Input: dimensioned drawing with shaded views. Units: mm. Origin: part minimum x, y, z. A direction names the side the tool comes from. Give positions to 0.01 mm unless a question says otherwise; leave off trailing zeros. Loops run counter-clockwise (first coordinate to the right, second up) from the corner with the lowest first, then second, coordinate; pieces in that order, holes last.
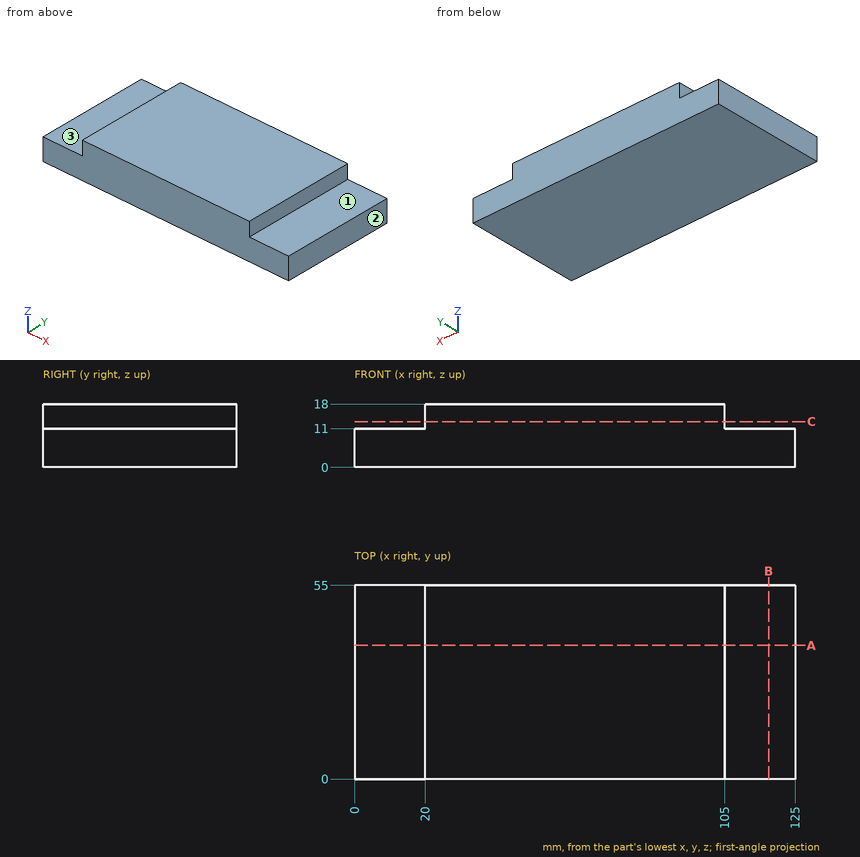
(1) Section C-C, the plane z = 13. Return the cut outline in (x, y), then the cut area to 4 significant figures.
A:
outline: (20, 0) - (105, 0) - (105, 55) - (20, 55) - close
area: 4,675 mm2
(2) Section B-B, the plane x = 117.5. Return the cut outline in (y, z).
A:
outline: (0, 0) - (55, 0) - (55, 11) - (0, 11) - close
(3) Section A-A, the plane y = 38. Return the cut outline in (x, z).
A:
outline: (0, 0) - (125, 0) - (125, 11) - (105, 11) - (105, 18) - (20, 18) - (20, 11) - (0, 11) - close
(4) Ray query, line 1 along X through (y, z) = (50.5, 13.25); line 2 along Z through (x, y) = (16.5, 23). Return the intervals inside material, ascending.
A:
line 1: x = 20 to 105
line 2: z = 0 to 11
(5) Reachability of the marked faces 1, 2 and 3 from +Z, -Z, +X, -X, +Y, -Y: full face, straight path, thin tool, end or side. Return the list, or none.
A:
face 1: +Z, +X, +Y, -Y
face 2: +Z, -Z, +X, +Y, -Y
face 3: +Z, -X, +Y, -Y
(6) First-contact query: pin 1 (1.5 mm diameter, centred on y = 17.5, z = 14.5, fed in from +X); pin 2 (3.5 mm diameter, centred on y = 40, z = 14, fed in from -X); pin 3 (6 mm diameter, centred on x = 120, y = 37.5, fed in from +Z). Flat tips, straight axial feed; report the tip coordinate or a pass-through.
A:
pin 1: stops at x = 105
pin 2: stops at x = 20
pin 3: stops at z = 11
